Read the model definition and answer for the solid it produces. Units are mm, in the model's axes. A direction names the side the tool comes from. Coordinates: 2 decimals unless noted, no trailing zeros. Write each loop counter-clockwise with the first axis right and the second up, starting at its lowest first coordinate (ties: lowest second). Pieces come first, ordered by that corner, then holes.
Item 1: Each of these flat-tipped pins is pushed along its axis until it touches: P1, Ø2.5, axis at y = 19.5, z = 5, coming from the +X side; P2, Ø2.5, axis at y = 19.5, z = 5, coming from the -X side; P3, Ø6, axis at x = -8.5, z = 6.5, coming from the +Y side; P4, Ø1.4, axis at x = 5.5, z = 5, coming from the -Y side. Where does it stop, or does it pass through?
Item 2: Section D-D (y = 31.75) is taken. Give the vertices of the cut face in (x, z), then the cut area to 3 significant figures.
Item 3: A tool of negligible diameter and unlimited length cuts with its end or side. For faces 4 (the face through (9.26, 22.81, 8.443)), 5 (the face through (13.656, 21, 5)), 6 (the face through (5, 10.656, 0)), from which of +Z, -Z, +X, -X, +Y, -Y can it reach the whole face along a straight path? Write none if from no direction.
Item 4: Section C-C (x = 21.5) is taken. Give the vertices of the cut face in (y, z), then the cut area to 3 significant figures.
Item 5: Straight lines are drawn through the part: probe 1 along Z at (x, y) = (5.5, 29.25); probe 2 along Z at (x, y) = (16, 27.5); probe 3 along Z at (x, y) = (27, 25). For each, find the intervals that lie inside material, in ascending order.
Item 6: Section A-A (y = 26.25) is taken. Give the vertices of the cut face in (x, z), then the cut area to 3 significant figures.
Item 7: Section B-B (x = 32.5) is taken. Give the vertices of the cut face in (y, z), then the cut area to 3 significant figures.
Item 8: Determine the mould class of faces 1 (the face through (5.766, 10.135, 22.386)), 2 (the face through (5, 21, -2.5)), 3 (the face through (-19.937, 21.256, -0.035)) for opening direction Z: released by +Z, released by -Z, zero draft, split by the parting line, or undercut.
from build123d import *

# Parameters (mm, degrees)
SKETCH1_W                = 70
SKETCH1_H                = 20
SKETCH1_R                = 2
BOSS_EXTRUDE1_DEPTH      = 2.5
BOSS_EXTRUDE2_DEPTH      = 5
BOSS_EXTRUDE3_DEPTH      = 5
BOSS_EXTRUDE3_DEPTH_BACK = 17
SKETCH6_R                = 15
SKETCH6_R_2              = 12
SKETCH10_R               = 15
BOSS_EXTRUDE4_DEPTH      = 3
SKETCH11_R               = 2.5
CUT_EXTRUDE1_DEPTH       = 3
FILLET1_R                = 3


with BuildPart() as part:
    # Sketch1 → Boss-Extrude1 (new, symmetric)
    with BuildSketch(Plane.XY):
        with Locations((5.655737705, 20.655737705)):
            Rectangle(SKETCH1_W, SKETCH1_H)
        with Locations((-21.844262295, 20.655737705)):
            Circle(SKETCH1_R, mode=Mode.SUBTRACT)
        with Locations((33.155737705, 20.655737705)):
            Circle(SKETCH1_R, mode=Mode.SUBTRACT)
    extrude(amount=BOSS_EXTRUDE1_DEPTH, both=True)

    # Sketch4 → Boss-Extrude2 (add)
    with BuildSketch(Plane.XY.offset(2.5)):
        Polygon((5.655737705, 24.655737705), (13.655737705, 24.655737705), (13.655737705, 16.655737705), (5.655737705, 16.655737705), (-2.344262295, 16.655737705), (-2.344262295, 24.655737705), align=None)
    extrude(amount=BOSS_EXTRUDE2_DEPTH)

    # Sketch6 → Boss-Extrude3 (add, two sides: drawn at the far end of the back side and taken through both)
    with BuildSketch(Plane(origin=(0, 16.655737705, 0), x_dir=(-1, 0, 0), z_dir=(0, -1, 0)).offset(-BOSS_EXTRUDE3_DEPTH_BACK)):
        with Locations(Location((-5.655737705, -19.888643818, 0), (0, 0, 90))):
            Circle(SKETCH6_R)
        with Locations(Location((-5.655737705, -19.888643818, 0), (0, 0, 90))):
            Circle(SKETCH6_R_2, mode=Mode.SUBTRACT)
    extrude(amount=BOSS_EXTRUDE3_DEPTH + BOSS_EXTRUDE3_DEPTH_BACK)

    # Sketch10 → Boss-Extrude4 (add)
    with BuildSketch(Plane.XZ.offset(-11.655737705)):
        with Locations(Location((5.655737705, 19.888643818, 0), (0, 0, 270))):
            Circle(SKETCH10_R)
    extrude(amount=BOSS_EXTRUDE4_DEPTH)

    # Sketch11 → Cut-Extrude1 (cut)
    with BuildSketch(Plane.XZ.offset(-8.655737705)):
        with Locations(Location((5.655737705, 19.888643818, 0), (0, 0, 270))):
            Circle(SKETCH11_R)
    extrude(amount=-CUT_EXTRUDE1_DEPTH, mode=Mode.SUBTRACT)

    # Fillet1
    fillet1_edges = [part.edges().sort_by_distance(p)[0] for p in [
        (5.655737705, 8.655737705, 34.888643818),
    ]]
    fillet(fillet1_edges, radius=FILLET1_R - 0.0001)  # a hair under: the kernel refuses the full size


solid = part.part
Established:
1. P1: stops at x = 13.66
1. P2: stops at x = -2.34
1. P3: passes through
1. P4: stops at y = 9.6
2. outline: circle Ø30 at (5.66, 19.89); hole circle Ø24 at (5.66, 19.89)
2. area: 254 mm2
3. face 4: +Y
3. face 5: +X, +Y, -Y
3. face 6: -Z, +X, -X, -Y
4. outline: (10.66, -2.5) - (30.66, -2.5) - (30.66, 2.5) - (10.66, 2.5) - close
4. area: 100 mm2
5. probe 1: z = -2.5 to 2.5, 4.89 to 7.89, 31.89 to 34.89
5. probe 2: z = -2.5 to 2.5, 9.03 to 13.81, 25.97 to 30.75
5. probe 3: z = -2.5 to 2.5
6. outline: (-29.34, -2.5) - (40.66, -2.5) - (40.66, 2.5) - (-29.34, 2.5) - close; circle Ø30 at (5.66, 19.89); hole circle Ø24 at (5.66, 19.89)
6. area: 604 mm2
7. outline: (10.66, -2.5) - (18.77, -2.5) - (18.77, 2.5) - (10.66, 2.5) - close; (22.55, -2.5) - (30.66, -2.5) - (30.66, 2.5) - (22.55, 2.5) - close
7. area: 81.1 mm2
8. face 1: undercut
8. face 2: released by -Z
8. face 3: zero draft
